```python
from build123d import *

# Parameters (mm, degrees)
RESSALTO_EXTRUS_O1_DEPTH = 2.5
FILETE1_R                = 0.1


with BuildPart() as part:
    # Esboço1 → Ressalto-extrusão1 (new body)
    with BuildSketch(Plane.XY):
        with BuildLine():
            ThreePointArc((0.822871292, 142.838341472), (1.555104339, 141.070574519), (3.322871292, 140.338341472))
            Line((3.322871292, 140.338341472), (84.322871292, 140.338341472))
            ThreePointArc((84.322871292, 140.338341472), (86.090638245, 141.070574519), (86.822871292, 142.838341472))
            Line((86.822871292, 142.838341472), (86.822871292, 161.838341472))
            ThreePointArc((86.822871292, 161.838341472), (86.090638245, 163.606108425), (84.322871292, 164.338341472))
            Line((84.322871292, 164.338341472), (83.422871292, 164.338341472))
            Line((83.422871292, 164.338341472), (83.422871292, 156.838341472))
            Line((83.422871292, 156.838341472), (80.922871292, 156.838341472))
            Line((80.922871292, 156.838341472), (80.922871292, 164.338341472))
            Line((80.922871292, 164.338341472), (6.722871292, 164.338341472))
            Line((6.722871292, 164.338341472), (6.722871292, 156.838341472))
            Line((6.722871292, 156.838341472), (4.222871292, 156.838341472))
            Line((4.222871292, 156.838341472), (4.222871292, 164.338341472))
            Line((4.222871292, 164.338341472), (3.322871292, 164.338341472))
            ThreePointArc((3.322871292, 164.338341472), (1.555104339, 163.606108425), (0.822871292, 161.838341472))
            Line((0.822871292, 161.838341472), (0.822871292, 142.838341472))
        make_face()
    extrude(amount=RESSALTO_EXTRUS_O1_DEPTH)

    # Filete1
    filete1_edges = [part.edges().sort_by_distance(p)[0] for p in [
        (86.090638245, 141.070574519, 2.5),
        (0.822871292, 152.338341472, 0),
        (1.555104339, 163.606108425, 0),
        (3.772871292, 164.338341472, 0),
        (86.822871292, 152.338341472, 2.5),
        (4.222871292, 160.588341472, 0),
        (5.472871292, 156.838341472, 0),
        (6.722871292, 160.588341472, 0),
        (43.822871292, 164.338341472, 0),
        (80.922871292, 160.588341472, 0),
        (82.172871292, 156.838341472, 0),
        (83.422871292, 160.588341472, 0),
        (83.872871292, 164.338341472, 0),
        (86.090638245, 163.606108425, 2.5),
        (86.090638245, 163.606108425, 0),
        (86.822871292, 152.338341472, 0),
        (86.090638245, 141.070574519, 0),
        (43.822871292, 140.338341472, 0),
        (1.555104339, 141.070574519, 0),
        (83.872871292, 164.338341472, 2.5),
        (4.222871292, 164.338341472, 1.25),
        (4.222871292, 156.838341472, 1.25),
        (83.422871292, 160.588341472, 2.5),
        (6.722871292, 156.838341472, 1.25),
        (6.722871292, 164.338341472, 1.25),
        (80.922871292, 164.338341472, 1.25),
        (80.922871292, 156.838341472, 1.25),
        (83.422871292, 156.838341472, 1.25),
        (83.422871292, 164.338341472, 1.25),
        (82.172871292, 156.838341472, 2.5),
        (80.922871292, 160.588341472, 2.5),
        (43.822871292, 164.338341472, 2.5),
        (6.722871292, 160.588341472, 2.5),
        (5.472871292, 156.838341472, 2.5),
        (1.555104339, 141.070574519, 2.5),
        (4.222871292, 160.588341472, 2.5),
        (3.772871292, 164.338341472, 2.5),
        (1.555104339, 163.606108425, 2.5),
        (0.822871292, 152.338341472, 2.5),
        (43.822871292, 140.338341472, 2.5),
    ]]
    fillet(filete1_edges, radius=FILETE1_R)


solid = part.part
```
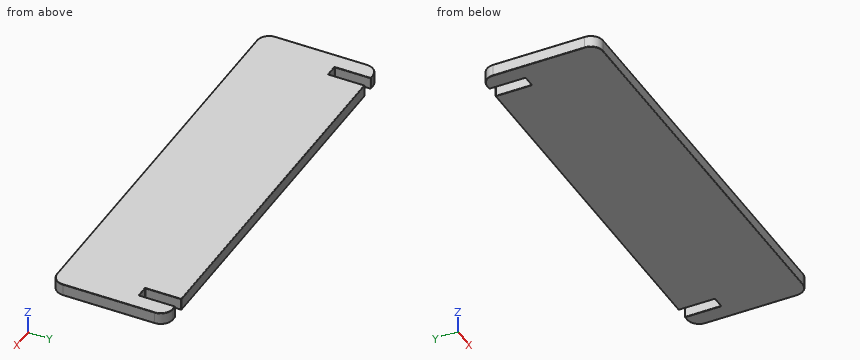
Source: CAD feature listing. Evaluate the final solid. Frame: model axes, mm. Give positions to 0.01 mm unless a question says otherwise; leave off trailing zeros. Loops run counter-clockwise (first coordinate to the right, second up) from the corner with the lowest first, then second, coordinate; pieces in that order, holes last. Notation, with made-up numbers: (33, 75.25) - (72, 75.25) arc R29 ccw to (72, 108.25) - close; hole circle Ø10 at (6, 39.5). An arc over 180 degrees is marked (long way). Use CSV: the item, a comma, the result in double quotes. Start each with the question number.
1. Section B-B (z = 1.1). Output: boundary loops of the cut face in (x, y), then the cut area to 3 significant figures.
2. Ray query, L1, parallel to X at y = 157.25, z = 0.95; L2, parallel to X at y = 162.25, z = 1.8; L3, parallel to Y at x = 82, z = 1.15. Return the intervals inside material, ascending.
3. Pin query (flat end, axial travel): pin 1 (1.5 mm diameter, centred on x = 12.5, y = 146, fed in from -Z). Return the tip coordinate at first contact, or that it passes through.
4. Section A-A (y = 160.25). Output: boundary loops of the cut face in (x, z).
Response:
1,outline,"(0.82, 142.84) arc R2.5 ccw to (3.32, 140.34) - (84.32, 140.34) arc R2.5 ccw to (86.82, 142.84) - (86.82, 161.84) arc R2.5 ccw to (84.32, 164.34) - (83.52, 164.34) arc R0.1 ccw to (83.42, 164.24) - (83.42, 156.94) arc R0.1 cw to (83.32, 156.84) - (81.02, 156.84) arc R0.1 cw to (80.92, 156.94) - (80.92, 164.24) arc R0.1 ccw to (80.82, 164.34) - (6.82, 164.34) arc R0.1 ccw to (6.72, 164.24) - (6.72, 156.94) arc R0.1 cw to (6.62, 156.84) - (4.32, 156.84) arc R0.1 cw to (4.22, 156.94) - (4.22, 164.24) arc R0.1 ccw to (4.12, 164.34) - (3.32, 164.34) arc R2.5 ccw to (0.82, 161.84) - close"
1,area,"2,020 mm²"
2,L1,"0.82 to 4.22, 6.72 to 80.92, 83.42 to 86.82"
2,L2,"0.86 to 4.22, 6.72 to 80.92, 83.42 to 86.79"
2,L3,"140.34 to 156.84"
3,pin 1,"z = 0"
4,outline,"(0.82, 0.1) arc R0.1 ccw to (0.92, 0) - (4.12, 0) arc R0.1 ccw to (4.22, 0.1) - (4.22, 2.4) arc R0.1 ccw to (4.12, 2.5) - (0.92, 2.5) arc R0.1 ccw to (0.82, 2.4) - close; (6.72, 0.1) arc R0.1 ccw to (6.82, 0) - (80.82, 0) arc R0.1 ccw to (80.92, 0.1) - (80.92, 2.4) arc R0.1 ccw to (80.82, 2.5) - (6.82, 2.5) arc R0.1 ccw to (6.72, 2.4) - close; (83.42, 0.1) arc R0.1 ccw to (83.52, 0) - (86.72, 0) arc R0.1 ccw to (86.82, 0.1) - (86.82, 2.4) arc R0.1 ccw to (86.72, 2.5) - (83.52, 2.5) arc R0.1 ccw to (83.42, 2.4) - close"
